Verification items for the finished model (mm, model axes). A direction names the side the tool comes from. Round coordinates to 2 decimals unless told otherwise and drop trailing zeros. Write each loop counter-clockwise with the first axis right and the second up, starting at its lowest first coordinate (ties: lowest second). Pieces come first, ordered by that corner, then holes. Notation, with made-up numbers: (49.5, 70) -> (53.5, 70) arc R17 cw to (53.5, 86) -> close; hole circle Ø6 at (-10.5, 34.25). An arc over 180 degrees is marked (long way). Answer as a JSON object with one key per item and string values. Group by question number.
(1) Gauge pin test, flat ends, axial feed: pin 1 Ø24 at (y, z) = (195, 150) entering from +X; pin 2 Ø6 at (x, z) = (2.5, 180) entering from -Y; pin 3 Ø20 at (x, y) = (39, 24) entering from -Z. Record the tip position at first contact, or that the pin passes through.
(2) Sectioned sample at A-A on z = 150. Record the cut outline in (x, y).
(3) Sectioned sample at C-C on y = 146. Record the cut outline in (x, z).
(4) Scan lines: L1, parallel to Y at x = 0, z = 150; L2, parallel to X at y = 71.5, z = 37.5; L3, parallel to Y at x = 3.5, z = 162. Record each from-to range of solid material in increasing order. Write a range as from..to.
(5) Draft check along Y on faces 6 (the face through (0, 20, -10)), 7 (the face through (-48.7, 20.3, -0.1)), 8 (the face through (-0.175, 197.253, 142.846)). Enter one of: released by +Y, released by -Y, zero draft, split by the parting line, or undercut.
(6) Set-up check for faces 1 (the face through (-1, 0, 0)), 2 (the face through (0, 110, 75)), 3 (the face through (0.18, 152.92, 187.15)), 4 (the face through (41, 15, -7.5)), 5 (the face through (-33, 11, -7.5)): record each of +Z, -Z, +X, -X, +Y, -Y from which the full face is reachable in a straight line by a thin tool's end or side.
(7) Sectioned sample at B-B on x = -9.5. Record the cut outline in (y, z), and give its area (3 significant figures).
(8) Sectioned sample at D-D on y = 30.5. Record the cut outline in (x, z).
```python
from build123d import *

# Parameters (mm, degrees)
SKETCH2_W                  = 25
SKETCH2_H                  = 5
SKETCH2_H_2                = 15
SKETCH2_W_2                = 73.5
BOSS_EXTRUDE3_DEPTH        = 40
CUT_EXTRUDE1_DEPTH         = 15
CUT_EXTRUDE3_DEPTH         = 25
SKETCH5_W                  = 25
SKETCH5_H                  = 25
BOSS_EXTRUDE4_DEPTH        = 12.5
BOSS_EXTRUDE4_DEPTH_BACK   = 12.5
BOSS_EXTRUDE4_2_DEPTH      = 12.5
BOSS_EXTRUDE4_2_DEPTH_BACK = 12.5
BOSS_EXTRUDE5_START        = -12.5
BOSS_EXTRUDE5_DEPTH        = 25
SKETCH9_W                  = 25
SKETCH9_H                  = 25
SKETCH9_R                  = 7.5
BOSS_EXTRUDE6_DEPTH        = 12.5
BOSS_EXTRUDE6_DEPTH_BACK   = 12.5
BOSS_EXTRUDE7_DEPTH        = 12.5
BOSS_EXTRUDE7_DEPTH_BACK   = 12.5
BOSS_EXTRUDE8_DEPTH        = 12.5
BOSS_EXTRUDE8_DEPTH_BACK   = 12.5
CUT_EXTRUDE4_REACH         = 100.5
SKETCH12_W                 = 25
SKETCH12_H                 = 25
CUT_EXTRUDE5_REACH         = 100.5


with BuildPart() as part:
    # Sketch2 → Boss-Extrude3 (new body)
    with BuildSketch(Plane(origin=(0, 0, 0), x_dir=(1, 0, 0), z_dir=(0, 1, 0))):
        with Locations((0, -10)):
            Rectangle(SKETCH2_W, SKETCH2_H)
        Rectangle(SKETCH2_W, SKETCH2_H_2)
        with Locations((0, 10)):
            Rectangle(SKETCH2_W, SKETCH2_H)
        with Locations((-49.25, 0)):
            Rectangle(SKETCH2_W_2, SKETCH2_H_2)
        with Locations((49.25, 0)):
            Rectangle(SKETCH2_W_2, SKETCH2_H_2)
    extrude(amount=BOSS_EXTRUDE3_DEPTH)

    # Sketch6 → Cut-Extrude1 (cut)
    with BuildSketch(Plane(origin=(0, 0, -7.5), x_dir=(-1, 0, 0), z_dir=(0, 0, -1))):
        Polygon((12.5, 40), (86, 0), (86, 40), align=None)
    cut_extrude1 = extrude(amount=-CUT_EXTRUDE1_DEPTH, mode=Mode.SUBTRACT)

    # Mirror1: Cut-Extrude1 across plane
    add(cut_extrude1.mirror(Plane(origin=(0, 0, 0), x_dir=(0, 0, 1), z_dir=(1, 0, 0))), mode=Mode.SUBTRACT)

    # Sketch7 → Cut-Extrude3 (cut)
    with BuildSketch(Plane.ZY.offset(12.5)):
        Polygon((-12.5, 40), (-7.5, 0), (-12.5, 0), align=None)
    cut_extrude3 = extrude(amount=-CUT_EXTRUDE3_DEPTH, mode=Mode.SUBTRACT)

    # Mirror2: Cut-Extrude3 across plane
    add(cut_extrude3.mirror(Plane.XY), mode=Mode.SUBTRACT)



with BuildPart() as body_2:
    # Sketch5 → Boss-Extrude4 (new body, two sides)
    with BuildSketch(Plane(origin=(0, 0, 0), x_dir=(0, 0, -1), z_dir=(1, 0, 0))) as boss_extrude4_sk:
        with Locations((-75, 110)):
            Rectangle(SKETCH5_W, SKETCH5_H)
    extrude(amount=BOSS_EXTRUDE4_DEPTH)
    extrude(boss_extrude4_sk.sketch, amount=-BOSS_EXTRUDE4_DEPTH_BACK)


with BuildPart() as body_3:
    # Sketch5 → Boss-Extrude4 2 (new body, two sides)
    with BuildSketch(Plane(origin=(0, 0, 0), x_dir=(0, 0, -1), z_dir=(1, 0, 0))) as boss_extrude4_2_sk:
        with Locations((-225, 110)):
            Rectangle(SKETCH5_W, SKETCH5_H)
    extrude(amount=BOSS_EXTRUDE4_2_DEPTH)
    extrude(boss_extrude4_2_sk.sketch, amount=-BOSS_EXTRUDE4_2_DEPTH_BACK)


with BuildPart() as part_1:
    add(part.part)

    add(body_2.part)  # Boss-Extrude5 merges body 2
    # Sketch8 → Boss-Extrude5 (add)
    with BuildSketch(Plane(origin=(0, 0, 0), x_dir=(0, 0, -1), z_dir=(1, 0, 0)).offset(BOSS_EXTRUDE5_START)):
        Polygon((-62.5, 97.5), (-12.5, 40), (12.5, 40), (-62.5, 122.5), align=None)
    extrude(amount=BOSS_EXTRUDE5_DEPTH)



with BuildPart() as body_3_2:
    # Sketch9 → Boss-Extrude6 (new body, two sides)
    with BuildSketch(Plane(origin=(0, 0, 0), x_dir=(0, 0, -1), z_dir=(1, 0, 0))) as boss_extrude6_sk:
        with Locations((-150, 195)):
            Rectangle(SKETCH9_W, SKETCH9_H)
        with Locations((-150, 195)):
            Circle(SKETCH9_R, mode=Mode.SUBTRACT)
    extrude(amount=BOSS_EXTRUDE6_DEPTH)
    extrude(boss_extrude6_sk.sketch, amount=-BOSS_EXTRUDE6_DEPTH_BACK)


with BuildPart() as part_2:
    add(part_1.part)

    add(body_3_2.part)  # Boss-Extrude7 merges body 3 2
    # Sketch10 → Boss-Extrude7 (add, two sides)
    with BuildSketch(Plane(origin=(0, 0, 0), x_dir=(0, 0, -1), z_dir=(1, 0, 0))) as boss_extrude7_sk:
        Polygon((-137.5, 182.5), (-87.5, 122.5), (-62.5, 122.5), (-137.5, 207.5), align=None)
    extrude(amount=BOSS_EXTRUDE7_DEPTH)
    extrude(boss_extrude7_sk.sketch, amount=-BOSS_EXTRUDE7_DEPTH_BACK)


    add(body_3.part)  # Boss-Extrude8 merges body 3
    # Sketch11 → Boss-Extrude8 (add, two sides)
    with BuildSketch(Plane(origin=(0, 0, 0), x_dir=(0, 0, -1), z_dir=(1, 0, 0))) as boss_extrude8_sk:
        Polygon((-162.5, 182.5), (-212.5, 122.5), (-237.5, 122.5), (-162.5, 207.5), align=None)
    extrude(amount=BOSS_EXTRUDE8_DEPTH)
    extrude(boss_extrude8_sk.sketch, amount=-BOSS_EXTRUDE8_DEPTH_BACK)

    # Sketch12 → Cut-Extrude4 (cut, up to next)
    with BuildSketch(Plane.ZY.offset(12.5), mode=Mode.PRIVATE) as cut_extrude4_sk1:
        with Locations((225, 110)):
            Rectangle(SKETCH12_W, SKETCH12_H)
    cut_extrude4_tool1 = extrude(cut_extrude4_sk1.sketch, amount=-CUT_EXTRUDE4_REACH, mode=Mode.PRIVATE) & part_2.part
    add(cut_extrude4_tool1.solids().sort_by_distance((-12.5, 110, 225))[0], mode=Mode.SUBTRACT)

    # Sketch13 → Cut-Extrude5 (cut, up to next)
    with BuildSketch(Plane.ZY.offset(12.5), mode=Mode.PRIVATE) as cut_extrude5_sk1:
        Polygon((87.5, 122.5), (62.5, 97.5), (87.5, 97.5), align=None)
    cut_extrude5_tool1 = extrude(cut_extrude5_sk1.sketch, amount=-CUT_EXTRUDE5_REACH, mode=Mode.PRIVATE) & part_2.part
    add(cut_extrude5_tool1.solids().sort_by_distance((-12.5, 105.833333, 79.166667))[0], mode=Mode.SUBTRACT)


solid = part_2.part
```
Computed values:
{
 "1": {"pin 1": "x = 12.5", "pin 2": "y = 157.9", "pin 3": "z = -7.5"},
 "2": {"outline": "(-12.5, 182.5) -> (12.5, 182.5) -> (12.5, 187.5) -> (-12.5, 187.5) -> close; (-12.5, 202.5) -> (12.5, 202.5) -> (12.5, 207.5) -> (-12.5, 207.5) -> close"},
 "3": {"outline": "(-12.5, 83.24) -> (12.5, 83.24) -> (12.5, 107.08) -> (-12.5, 107.08) -> close; (-12.5, 192.92) -> (12.5, 192.92) -> (12.5, 216.76) -> (-12.5, 216.76) -> close"},
 "4": {"L1": "182.5..187.5, 202.5..207.5", "L2": "-12.5..12.5", "L3": "182.5..207.5"},
 "5": {"face 6": "released by -Y", "face 7": "released by +Y", "face 8": "undercut"},
 "6": {"face 1": "+Z, -Z, +X, -X, -Y", "face 2": "+Z, +X, -X, -Y", "face 3": "+X, -X, -Y", "face 4": "-Z, +X, +Y, -Y", "face 5": "-Z, -X, +Y, -Y"},
 "7": {"outline": "(0, -7.5) -> (40, -12.5) -> (122.5, 62.5) -> (207.5, 137.5) -> (207.5, 162.5) -> (122.5, 237.5) -> (122.5, 212.5) -> (182.5, 162.5) -> (182.5, 137.5) -> (122.5, 87.5) -> (97.5, 62.5) -> (40, 12.5) -> (0, 7.5) -> close; hole circle Ø15 at (195, 150)", "area": "6,590 mm2"},
 "8": {"outline": "(-29.96, -7.5) -> (-12.5, -7.5) -> (-12.5, -11.31) -> (12.5, -11.31) -> (12.5, -7.5) -> (29.96, -7.5) -> (29.96, 7.5) -> (12.5, 7.5) -> (12.5, 11.31) -> (-12.5, 11.31) -> (-12.5, 7.5) -> (-29.96, 7.5) -> close"}
}
